Source: CAD feature listing. Evaluate the final solid. Frame: model axes, mm. A direction names the side the tool comes from. Coordinates: 2 decimals unless noted, no trailing zeros. Order: outer loops, then holes, each group sorted by start corner. A loop starts at its lowest first (then second) coordinate and runs counter-clockwise, first axis right, second up.
```python
from build123d import *

# Parameters (mm, degrees)
BOX005_W      = 20
BOX005_H      = 317
BOX005_DEPTH  = 13.5
BOX004_W      = 20
BOX004_H      = 317
BOX004_DEPTH  = 15
SKETCH006_R   = 2.05
HOLE001_DEPTH = 638.969553
SKETCH008_R   = 2.05
HOLE003_DEPTH = 637.469553


with BuildPart() as cut016:
    # Box005 → Box005 (new body)
    with BuildSketch(Plane(origin=(1.5, 0, 1.5), x_dir=(1, 0, 0), z_dir=(0, 0, 1))):
        with Locations((10, 158.5)):
            Rectangle(BOX005_W, BOX005_H)
    extrude(amount=BOX005_DEPTH)


with BuildPart() as side_bottom_body:
    # Box004 → Box004 (new body)
    with BuildSketch(Plane.XY):
        with Locations((10, 158.5)):
            Rectangle(BOX004_W, BOX004_H)
    extrude(amount=BOX004_DEPTH)

    # Cut002: cut Cut016
    add(cut016.part, mode=Mode.SUBTRACT)


with BuildPart() as side_bottom_body_1:
    # Cut002 placement: moved
    add(side_bottom_body.part.moved(Location((1.5, 1.5, 21.5))))


with BuildPart() as side_bottom_body_2:
    # BaseFeature001 placement: moved
    add(side_bottom_body_1.part.moved(Location((-1.5, -1.5, -21.5))))

    # Sketch006 → Hole001 (cut, through all)
    with BuildSketch(Plane.YZ.offset(3)):
        with Locations((9.25, 8.25)):
            Circle(SKETCH006_R)
    hole001 = extrude(amount=-HOLE001_DEPTH, mode=Mode.SUBTRACT)

    # Mirrored: Hole001 across Sketch006 Axis0
    add(hole001.mirror(Plane(origin=(3, 158.5, 15), x_dir=(1, 0, 0), z_dir=(0, 1, 0))), mode=Mode.SUBTRACT)

    # Sketch008 → Hole003 (cut, through all)
    with BuildSketch(Plane.XY.offset(1.5)):
        with Locations((10.75, 10.75)):
            Circle(SKETCH008_R)
    hole003 = extrude(amount=-HOLE003_DEPTH, mode=Mode.SUBTRACT)

    # Mirrored001: Hole003 across Sketch008 Axis0
    add(hole003.mirror(Plane(origin=(20, 158.5, 1.5), x_dir=(0, 0, 1), z_dir=(0, -1, 0))), mode=Mode.SUBTRACT)


with BuildPart() as side_bottom_body_3:
    # Body001 placement: moved
    add(side_bottom_body_2.part.moved(Location((1.5, 1.5, 20))))


with BuildPart() as left_bottom_mirror:
    # Part__Mirroring001: instance of side_bottom_body
    add(side_bottom_body_3.part.mirror(Plane(origin=(2e-06, 160, 27.5), x_dir=(0, -1, 0), z_dir=(1, 0, 0))))


with BuildPart() as left_bottom_mirror_1:
    # Part__Mirroring001 placement: moved
    add(left_bottom_mirror.part.moved(Location((640, 0, 0))))


solid = left_bottom_mirror_1.part
```
Q1. Section query A-A on y = 276.5. Output: boundary loops of the cut face in (x, z).
Solutions:
outline: (618.5, 20) - (638.5, 20) - (638.5, 35) - (637, 35) - (637, 21.5) - (618.5, 21.5) - close
Q2. Set-up query: faces 4 (the flat face through (637, 158, 28)), 5 (the flat face through (638.5, 158, 27)). Return all of +Z, -Z, +X, -X, +Y, -Y with unobstructed straight access to the full face (end or side cutting, diameter ignored); none if empty.
Solutions:
face 4: +Z, -X, +Y, -Y
face 5: +Z, -Z, +X, +Y, -Y
Q3. Pull-direction query (Z, two-part tool) for faces 1 (the flat face through (628, 162, 21.5)), 2 (the flat face through (633, 1.5, 21)), 3 (the flat face through (629, 162, 20)); classes: pulls with the +Z half, pulls with the -Z half, needs draft (parallel to the pull), parting line crosses it, or undercut.
Solutions:
face 1: pulls with the +Z half
face 2: needs draft
face 3: pulls with the -Z half
Q4. Section query B-B on x = 622.5. Output: boundary loops of the cut face in (y, z).
Solutions:
outline: (1.5, 20) - (318.5, 20) - (318.5, 21.5) - (1.5, 21.5) - close
Q5. Pin query (flat end, axial travel): P1, Ø5.5, axis at y = 10.75, z = 28.25, coming from the -X side; P2, Ø9, axis at x = 625.5, y = 210.5, coming from the +Z side. Return the tip coordinate at first contact, or that it passes through.
Solutions:
P1: stops at x = 637
P2: stops at z = 21.5
Q6. Material intervals for line 1 along Z through (x, y) = (638, 10.75); line 2 along X through (y, z) = (307.75, 20.65); line 3 along X through (y, z) = (191, 22), sorted ascending.
Solutions:
line 1: z = 20 to 26.2, 30.3 to 35
line 2: x = 618.5 to 625.7, 629.8 to 638.5
line 3: x = 637 to 638.5
